The listing builds one solid part. Answer for the finished solid, in the listing's coordinates (mm). Face numbers are marked on the shaded views. A direction names the side the tool comes from. Round coordinates to 2 decimals unless told otherwise and drop trailing zeros. Loops run counter-clockwise (first coordinate to the right, second up) from the corner with the lowest first, then second, coordinate; pieces in that order, holes last. Notation, with made-up numbers: (-30.5, -13.75) -> (11.5, -13.75) arc R9 cw to (11.5, -3.75) -> close; hole circle Ø4 at (-10.75, 71). An arc over 180 degrees is marked (long way). Write each question's results on one line, items separated by ' | '. Start each with the question number.
(1) For the marked faces 1, 2 and 3, determine the directions among +Z, -Z, +X, -X, +Y, -Y from which every point of the face is accessible in a straight line to the end or side of a thin tool.
(2) The part is cut by section B-B (y = -2.5). Determine the outline of the cut face in (x, z), plus the area to 3 significant figures.
(3) The part is cut by section A-A (x = 2.45). Determine the outline of the cut face in (y, z), plus the area to 3 significant figures.
(4) Straight lines are drawn through the part: probe 1 along Z at (x, y) = (2.65, 0); probe 2 along Y at (x, z) = (2.4, 0); probe 3 along X at (y, z) = (-0.75, 0). For each, find the intervals that lie inside material, in ascending order.
(5) Determine the mould class of the marked faces 4, 5, 6 and 7 for opening direction Y: released by +Y, released by -Y, zero draft, split by the parting line, or undercut.
(6) The part is cut by section D-D (y = 3.25). Determine the outline of the cut face in (x, z).
(7) The part is cut by section C-C (z = 0). Determine the outline of the cut face in (x, y), plus the area to 3 significant figures.
(8) Flat-ended cylindrical pins translate along their axes: pin 1 (0.8 mm diameter, centred on x = 2.5, y = 4, fed in from +Z); pin 2 (3.5 mm diameter, centred on y = 0, z = 0, fed in from +X). Find the tip coordinate at first contact, or state that the pin passes through.
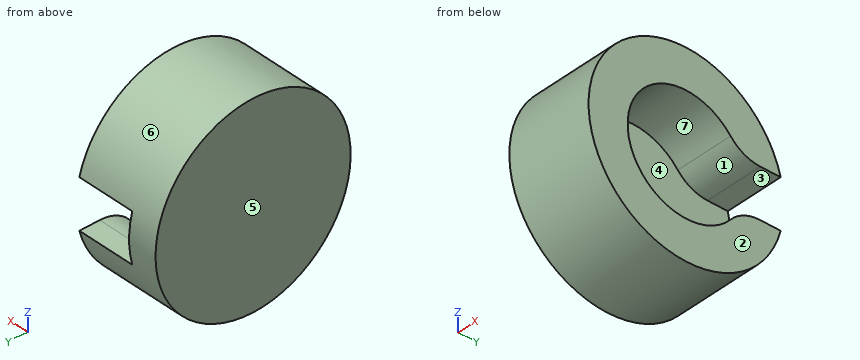
```python
from build123d import *

# Parameters (mm, degrees)
SKETCH1_R           = 5
BOSS_EXTRUDE1_DEPTH = 1.5
SKETCH2_R           = 5
SKETCH2_R_2         = 3
BOSS_EXTRUDE2_DEPTH = 3
CUT_EXTRUDE1_DEPTH  = 8.681145748
FILLET1_R           = 2


with BuildPart() as part:
    # Sketch1 → Boss-Extrude1 (new body)
    with BuildSketch(Plane(origin=(0, 0, 0), x_dir=(0, 0, -1), z_dir=(1, 0, 0))):
        Circle(SKETCH1_R)
    extrude(amount=BOSS_EXTRUDE1_DEPTH)

    # Sketch2 → Boss-Extrude2 (add)
    with BuildSketch(Plane(origin=(1.5, 0, 0), x_dir=(0, 0, -1), z_dir=(1, 0, 0))):
        Circle(SKETCH2_R)
        Circle(SKETCH2_R_2, mode=Mode.SUBTRACT)
    extrude(amount=BOSS_EXTRUDE2_DEPTH)

    # Sketch3 → Cut-Extrude1 (cut, through all)
    with BuildSketch(Plane(origin=(1.5, 0, 0), x_dir=(0, 0, -1), z_dir=(1, 0, 0))):
        with BuildLine():
            Line((-1.25, 6), (-1.25, 2.727178029))
            ThreePointArc((-1.25, 2.727178029), (0, 3), (1.25, 2.727178029))
            Line((1.25, 2.727178029), (1.25, 6))
            Line((1.25, 6), (-1.25, 6))
        make_face()
        with BuildLine():
            Line((-1.25, 2.727178029), (-1.25, 0))
            Line((-1.25, 0), (1.25, 0))
            Line((1.25, 0), (1.25, 2.727178029))
            ThreePointArc((1.25, 2.727178029), (0, 3), (-1.25, 2.727178029))
        make_face()
        with BuildLine():
            Line((1.25, 0), (-1.25, 0))
            Line((-1.25, 0), (-1.25, -2.727178029))
            ThreePointArc((-1.25, -2.727178029), (0, -3), (1.25, -2.727178029))
            Line((1.25, -2.727178029), (1.25, 0))
        make_face()
    extrude(amount=CUT_EXTRUDE1_DEPTH, mode=Mode.SUBTRACT)

    # Fillet1
    fillet1_edges = [part.edges().sort_by_distance(p)[0] for p in [
        (3, 2.727178029, 1.25),
        (3, 2.727178029, -1.25),
    ]]
    fillet(fillet1_edges, radius=FILLET1_R)


solid = part.part
```
Checked values:
1) face 1: +X | face 2: +Z, -Z, +X, +Y, -Y | face 3: +X, +Y
2) outline: (0, -4.33) -> (4.5, -4.33) -> (4.5, -1.66) -> (1.5, -1.66) -> (1.5, 1.66) -> (4.5, 1.66) -> (4.5, 4.33) -> (0, 4.33) -> close | area: 29.0 mm2
3) outline: (2.28, -1.95) arc R3 cw (long way) to (2.28, 1.95) arc R2 ccw to (3.8, 1.25) -> (4.84, 1.25) arc R5 ccw (long way) to (4.84, -1.25) -> (3.8, -1.25) arc R2 ccw to start | area: 44.9 mm2
4) probe 1: z = -5 to -3, 3 to 5 | probe 2: y = -5 to -3 | probe 3: x = 0 to 1.5
5) face 4: undercut | face 5: zero draft | face 6: split by the parting line | face 7: undercut
6) outline: (0, -3.8) -> (4.5, -3.8) -> (4.5, -1.33) -> (1.5, -1.33) -> (1.5, 1.33) -> (4.5, 1.33) -> (4.5, 3.8) -> (0, 3.8) -> close
7) outline: (0, -5) -> (4.5, -5) -> (4.5, -3) -> (1.5, -3) -> (1.5, 5) -> (0, 5) -> close | area: 21.0 mm2
8) pin 1: stops at z = 3.47 | pin 2: stops at x = 1.5
